from build123d import *

# Parameters (mm, degrees)
F0_W      = 62
F0_H      = 15
F1_DEPTH  = 50
F3_DEPTH  = 20
F7_DEPTH  = 62
F8_DEPTH  = 9
F10_DEPTH = 25


# Not quite as in the source:
# - a pattern or mirror of a feature is missing from the dataset's text; its kind, count and spacing are read off the source's solid


with BuildPart() as f1:
    # F0 (on Front) → F1 (new body)
    with BuildSketch(Plane.XZ):
        with Locations((0, 7.5)):
            Rectangle(F0_W, F0_H)
    extrude(amount=F1_DEPTH)

    # F2 (on face) → F3 (join)
    with BuildSketch(Plane(origin=(0, 0, 0), x_dir=(-1, 0, 0), z_dir=(0, 1, 0))):
        Polygon((-31, 15), (31, 15), (31, 42), (15, 42), (0, 27), (-15, 42), (-31, 42), align=None)
    extrude(amount=-F3_DEPTH)

    # F5 (on face) → F7 (cut)
    with BuildSketch(Plane(origin=(-31, 0, 0), x_dir=(0, -1, 0), z_dir=(-1, 0, 0))):
        Polygon((16, 6), (16, 0), (25, 0), (34, 0), (34, 6), align=None)
    extrude(amount=-F7_DEPTH, mode=Mode.SUBTRACT)

    # F6 (on face) → F8 (join)
    with BuildSketch(Plane(origin=(-31, 0, 0), x_dir=(0, -1, 0), z_dir=(-1, 0, 0))):
        Polygon((50, 15), (20, 42), (20, 15), align=None)
    f8 = extrude(amount=-F8_DEPTH)

    # F8_copies: F8 across plane
    add(f8.mirror(Plane(origin=(0, 0, 0), x_dir=(0, 0, 1), z_dir=(1, 0, 0))))

    # F9 (on face) → F10 (cut)
    with BuildSketch(Plane.XY.offset(15)):
        Polygon((0, -44), (-9, -50), (9, -50), align=None)
    extrude(amount=-F10_DEPTH, mode=Mode.SUBTRACT)


solid = f1.part
Build history of the part. All positions in model axes, mm. A direction names the side the tool comes from. Give positions to 0.01 mm unless a question says otherwise; leave off trailing zeros. Order: outer loops, then holes, each group sorted by start corner. A loop starts at its lowest first (then second) coordinate and runs counter-clockwise, first axis right, second up. Notation, with made-up numbers: M 66.5,88 L 87.5,88 A22 cw 87.5,96 Z; hole C 65.25,-25 d7. An arc over 180 degrees is marked long. Put each result on its own line as item: value.
Item 1: Probe line 1 (Y direction, x = 15, z = 3); line 2 (X direction, y = -36, z = 25.5); line 3 (Y direction, x = 15.5, z = 17.5). List the from-to ranges inside material, lowest first. Write a range as [from, to].
From the geometry:
line 1: y = [-50, -34], [-16, 0]
line 2: x = [-31, -22], [22, 31]
line 3: y = [-20, 0]
Item 2: Flat gauge pins, fed straight in: pin 1 Ø6 at (x, y) = (11.5, -25) entering from -Z; pin 2 Ø2 at (x, y) = (21.5, -26) entering from +Z; pin 3 Ø9 at (x, y) = (1, -31) entering from +Z. Where does each tip first touch, or does it go through?
From the geometry:
pin 1: stops at z = 6
pin 2: stops at z = 37.38
pin 3: stops at z = 15
Item 3: Two-plate mould, pull along Y, no slides. Class faces 5 (the flat face through (23, -10, 42)), 6 (the flat face through (0, -16, 3)), 7 (the flat face through (26.56, -35.21, 28.31)): +Y half, -Y half, draft (parallel to the pull), parting line (faces both ways), or undercut.
From the geometry:
face 5: draft
face 6: undercut
face 7: -Y half
Item 4: Slice it at C-C, the plane y = -40. Write the cut outline in (x, z), plus the area to 3 significant figures.
From the geometry:
outline: M -31,0 L 31,0 L 31,24 L 22,24 L 22,15 L -22,15 L -22,24 L -31,24 Z
area: 1,090 mm2
Item 5: 3-axis set-ups, long thin cutter, end or side, ignore diameter. For faces 1 (the flat face through (0, -34, 3)), 2 (the flat face through (-8, -10, 35)), 3 (the flat face through (4.56, -47.04, 7.6)), 4 (the flat face through (-22, -28, 23)): which of +Z, -Z, +X, -X, +Y, -Y reach the whole face in a straight line?
From the geometry:
face 1: -Z, +X, -X
face 2: +Z, +Y, -Y
face 3: +Z, -Z, -Y
face 4: +Z, -Y
Item 6: Slice it at D-D, the plane z = 38. Write the cut outline in (x, y).
From the geometry:
outline: M -31,-24.44 L -22,-24.44 L -22,-20 L -11,-20 L -11,0 L -31,0 Z; M 11,-20 L 22,-20 L 22,-24.44 L 31,-24.44 L 31,0 L 11,0 Z
Item 7: Slice it at A-A, the plane y = -45. Write the cut outline in (x, z), plus the area to 3 significant figures.
From the geometry:
outline: M -31,0 L -1.5,0 L -1.5,15 L -22,15 L -22,19.5 L -31,19.5 Z; M 1.5,0 L 31,0 L 31,19.5 L 22,19.5 L 22,15 L 1.5,15 Z
area: 966 mm2
Item 8: Slice it at B-B, the plane x = -7.5. Write the cut outline in (y, z), plus the area to 3 significant figures.
From the geometry:
outline: M -49,0 L -34,0 L -34,6 L -16,6 L -16,0 L 0,0 L 0,34.5 L -20,34.5 L -20,15 L -49,15 Z
area: 1,020 mm2
